Geometry: final body of the model. Coordinates: model frame, mm. A direction names the side the tool comes from. Give positions to 0.01 mm unless a question says otherwise; leave off trailing zeros. Order: outer loops, then holes, each group sorted by start corner. A loop starts at its lowest first (then second) coordinate and runs counter-clockwise, first axis right, second up. Notation, with made-up numbers: (57.25, 82) -> (64.25, 82) arc R21 cw to (64.25, 90) -> close; hole circle Ø5 at (-7, 61). An arc over 180 degrees is marked (long way). Answer in a Markdown table with one row per item. Add a question column.
Q1. Cut plane D-D on y = -7.5. Return the cut outline in (x, z), and give its area (3 significant figures).
Q2. Set-up query: faces 1 (the face through (8, -10.269, 1)), 2 (the face through (2, -12, 1)), 3 (the face through (2, 0, 1)). Return all of +Z, -Z, +X, -X, +Y, -Y with unobstructed straight access to the full face (end or side cutting, diameter ignored); none if empty.
Q3. Cut plane B-B on z = 0.9. Return the cut outline in (x, y).
Q4. Contact query for a flat-ended pin moving along its axis: P1, Ø0.6, axis at x = 1.5, z = 1, coming from the +Y side. Output: stop coordinate, or through.
Q5. Line query: line 1 along X through (y, z) = (-6.75, 1.2); line 2 along Y through (x, z) = (3.25, 1.65); line 3 along X through (y, z) = (-16.5, 0.9). Output: solid intervals per line, ascending. Write a range as from..to.
Q6. Pull-direction query (Y, two-part tool) for faces 4 (the face through (12, -10.269, 1)), 5 (the face through (10, -25, 1)), 6 (the face through (0, -6, 1)); classes: +Y half, -Y half, draft (parallel to the pull), parting line (faces both ways), or undercut.
Q7. Cut plane A-A on y = -13.5. Return the cut outline in (x, z).
Q8. Cut plane C-C on x = 1. Return the cut outline in (y, z), and give its area (3 significant figures).
from build123d import *

# Parameters (mm, degrees)
EXTRUDE_1_DEPTH     = 2
CUT_EXTRUDE_1_DEPTH = 2
FILLET_1_R          = 3


with BuildPart() as part:
    # ｽｹｯﾁ1 → ﾎﾞｽ - 押し出し1 (new body)
    with BuildSketch(Plane.XY):
        Polygon((4, 0), (0, 0), (0, -12), (4, -12), (4, -25), (16, -25), (16, 3), (4, 3), align=None)
    extrude(amount=EXTRUDE_1_DEPTH)

    # ｽｹｯﾁ2 → ｶｯﾄ - 押し出し1 (cut)
    with BuildSketch(Plane.XY.offset(2)):
        Polygon((11.632823949, -5.570087609), (8.772941266, -5.570087609), (8.772941266, -10.268637818), (7.260776917, -10.268637818), (10.202882607, -14.99997105), (13.144988298, -10.268637818), (11.632823949, -10.268637818), align=None)
    extrude(amount=-CUT_EXTRUDE_1_DEPTH, mode=Mode.SUBTRACT)

    # ﾌｨﾚｯﾄ1
    fillet_1_edges = [part.edges().sort_by_distance(p)[0] for p in [
        (16, 3, 1),
    ]]
    fillet(fillet_1_edges, radius=FILLET_1_R)


solid = part.part
Completed:
| question | item | result |
|---|---|---|
| 1 | outline | (0, 0) -> (8.77, 0) -> (8.77, 2) -> (0, 2) -> close; (11.63, 0) -> (16, 0) -> (16, 2) -> (11.63, 2) -> close |
| 1 | area | 26.3 mm² |
| 2 | face 1 | +Z, -Z |
| 2 | face 2 | +Z, -Z, -X, -Y |
| 2 | face 3 | +Z, -Z, -X, +Y |
| 3 | outline | (0, -12) -> (4, -12) -> (4, -25) -> (16, -25) -> (16, 0) arc R3 ccw to (13, 3) -> (4, 3) -> (4, 0) -> (0, 0) -> close; hole (7.26, -10.27) -> (10.2, -15) -> (13.14, -10.27) -> (11.63, -10.27) -> (11.63, -5.57) -> (8.77, -5.57) -> (8.77, -10.27) -> close |
| 4 | P1 | stops at y = 0 |
| 5 | line 1 | x = 0..8.77, 11.63..16 |
| 5 | line 2 | y = -12..0 |
| 5 | line 3 | x = 4..16 |
| 6 | face 4 | undercut |
| 6 | face 5 | -Y half |
| 6 | face 6 | draft |
| 7 | outline | (4, 0) -> (9.27, 0) -> (9.27, 2) -> (4, 2) -> close; (11.14, 0) -> (16, 0) -> (16, 2) -> (11.14, 2) -> close |
| 8 | outline | (-12, 0) -> (0, 0) -> (0, 2) -> (-12, 2) -> close |
| 8 | area | 24.0 mm² |
